Work out the finished part from the listing and answer in its coordinate system (mm). Round coordinates to 2 decimals unless told otherwise and drop trailing zeros. Write each loop counter-clockwise with the first axis right and the second up, starting at its lowest first coordinate (ties: lowest second). Pieces come first, ordered by that corner, then holes. Notation, with made-up numbers: (60, -28) -> (83, -28) arc R22 ccw to (83, -10) -> close; hole circle Ø4 at (-23.75, 61.5). An arc over 180 degrees is marked (long way). One line per item, written item: value.
```python
from build123d import *

# Parameters (mm, degrees)
SKETCH1_R                   = 18.25625
BOSS_EXTRUDE1_DEPTH         = 120.65
CHAMFER1_SIZE               = 5.55625
CHAMFER1_SIZE2              = 25.4
F_1_4_20_TAPPED_HOLE1_D     = 5.1054
F_1_4_20_TAPPED_HOLE1_DEPTH = 16.51
F_1_4_20_TAPPED_HOLE1_TIP   = 1.533816902


with BuildPart() as part:
    # Sketch1 → Boss-Extrude1 (new body)
    with BuildSketch(Plane(origin=(0, 0, 0), x_dir=(1, 0, 0), z_dir=(0, 1, 0))):
        Circle(SKETCH1_R)
    extrude(amount=BOSS_EXTRUDE1_DEPTH)

    # Chamfer1
    chamfer1_edges = [part.edges().sort_by_distance(p)[0] for p in [
        (-18.25625, 0, 0),
    ]]
    chamfer1_side = [part.faces().sort_by_distance(p)[0] for p in [
        (0, 0, 0),
    ]]
    chamfer(chamfer1_edges, length=CHAMFER1_SIZE, length2=CHAMFER1_SIZE2, reference=chamfer1_side[0])

    # 1/4-20 Tapped Hole1
    with Locations(Plane(origin=(0, 120.65, 0), x_dir=(1, 0, 0), z_dir=(0, 1, 0))):
        with Locations((0, 0)):
            Hole(F_1_4_20_TAPPED_HOLE1_D / 2, depth=F_1_4_20_TAPPED_HOLE1_DEPTH)
            with Locations((0, 0, -(F_1_4_20_TAPPED_HOLE1_DEPTH + F_1_4_20_TAPPED_HOLE1_TIP / 2))):  # 118° drill point
                Cone(0, F_1_4_20_TAPPED_HOLE1_D / 2, F_1_4_20_TAPPED_HOLE1_TIP, mode=Mode.SUBTRACT)


solid = part.part
```
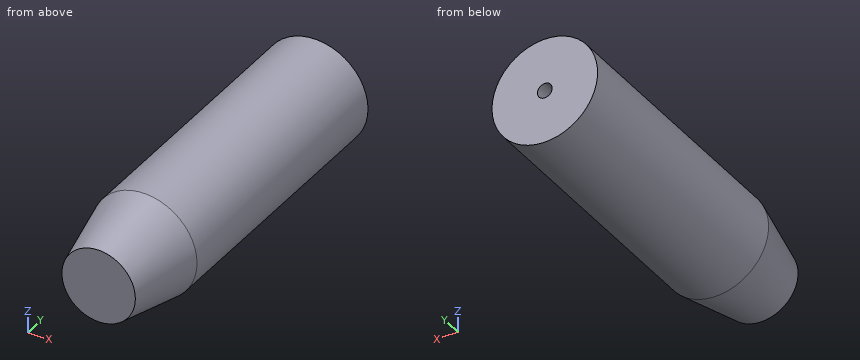
(1) Find section A-A on y = 17. Give the vertices of the cut face in (x, z), plus the area to 3 significant figures.
Reported:
outline: circle Ø32.84 at (0, 0)
area: 847 mm2
(2) Flat-ended cylindrical pins translate along their axes: pin 1 Ø1.5 at (y, z) = (90, -14.5) entering from -X; pin 2 Ø3 at (x, y) = (11.5, 59.5) entering from +Z; pin 3 Ø8 at (y, z) = (35.5, -14) entering from +X. Find the tip coordinate at first contact, or state that the pin passes through.
Reported:
pin 1: stops at x = -12.01
pin 2: stops at z = 15.27
pin 3: stops at x = 15.27
(3) Consider probe 1 along Z at (x, y) = (0, 111); probe 2 along X at (y, z) = (105.5, -1); probe 3 along X at (y, z) = (86.5, 12). Determine where each line is inside the solid, lowest interval first.
Reported:
probe 1: z = -18.26 to -2.55, 2.55 to 18.26
probe 2: x = -18.23 to -2.35, 2.35 to 18.23
probe 3: x = -13.76 to 13.76
